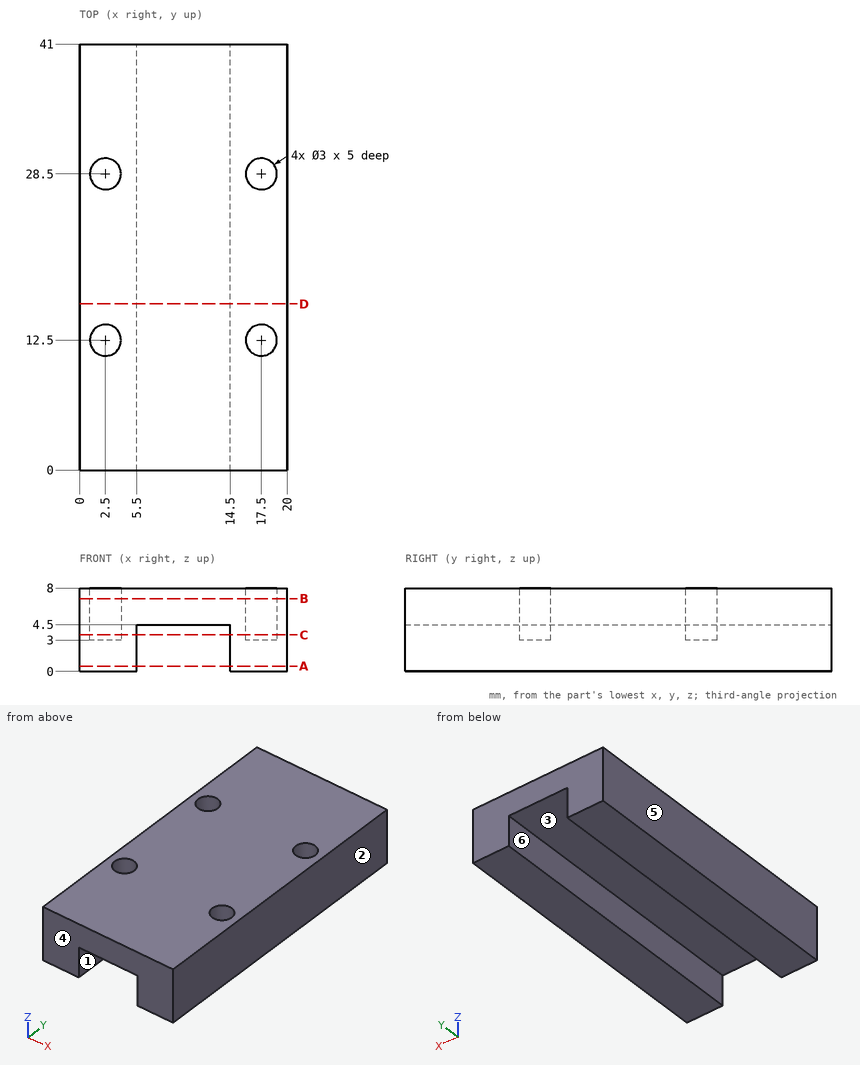
Part print with two shaded views. Sizes in mm from the minimum x, y, z corner. A direction names the side the tool comes from. Round coordinates to 2 decimals unless told otherwise and drop trailing zeros. Order: outer loops, then holes, each group sorted by start corner. A loop starts at its lowest first (then second) coordinate and runs counter-clockwise, first axis right, second up. Notation, with made-up numbers: M -26,71.25 L -22,71.25 A17 cw -22,91.25 Z; hole C 41.25,86.25 d6. An arc over 180 degrees is marked long. Answer in a Markdown table with one row per item. Add a question column.
Q1. Pin check, flat tips, straight feed: pin 1 (1.5 mm diameter, centred on x = 17, y = 28.5, fed in from +Z); pin 2 (1 mm diameter, centred on x = 13, z = 2, fed in from -Y); pin 3 (7 mm diameter, centred on x = 10, y = 15, fed in from -Z). Stop position of each tip, or through.
Q2. Cut at D-D on y = 16. Give the cut face in (x, z), and give its area (4 significant figures).
Q3. Mould opens along X. For the marked faces 3, 4, 5 and 6 say: +X half, -X half, draft (parallel to the pull), parting line (faces both ways), or undercut.
Q4. Cut at B-B on z = 7. Give the cut face in (x, y), and give its area (3 significant figures).
Q5. 3-axis set-ups, long thin cutter, end or side, ignore diameter. For the marked faces 1 and 2: which of +Z, -Z, +X, -X, +Y, -Y reach the whole face in a straight line?
Q6. Cut at C-C on z = 3.5. Give the cut face in (x, y), and give its area (3 significant figures).
Q7. Wall check: L1, parallel to Y at x = 17.5, z = 4.25; L2, parallel to X at y = 25, z = 3; L3, parallel to Y at x = 2, z = 6.5. Give the ranges that are in metal, low to high. Write a range as from..to.
Q8. Cut at A-A on z = 0.5. Give the cut face in (x, y), and give its area (3 significant figures).
Established:
| question | item | result |
|---|---|---|
| 1 | pin 1 | stops at z = 3 |
| 1 | pin 2 | passes through |
| 1 | pin 3 | stops at z = 4.5 |
| 2 | outline | M 0,0 L 5.5,0 L 5.5,4.5 L 14.5,4.5 L 14.5,0 L 20,0 L 20,8 L 0,8 Z |
| 2 | area | 119.5 mm2 |
| 3 | face 3 | undercut |
| 3 | face 4 | draft |
| 3 | face 5 | -X half |
| 3 | face 6 | undercut |
| 4 | outline | M 0,0 L 20,0 L 20,41 L 0,41 Z; hole C 2.5,12.5 d3; hole C 2.5,28.5 d3; hole C 17.5,12.5 d3; hole C 17.5,28.5 d3 |
| 4 | area | 792 mm2 |
| 5 | face 1 | -Z, +Y, -Y |
| 5 | face 2 | +Z, -Z, +X, +Y, -Y |
| 6 | outline | M 0,0 L 5.5,0 L 5.5,41 L 0,41 Z; M 14.5,0 L 20,0 L 20,41 L 14.5,41 Z; hole C 2.5,12.5 d3; hole C 2.5,28.5 d3; hole C 17.5,12.5 d3; hole C 17.5,28.5 d3 |
| 6 | area | 423 mm2 |
| 7 | L1 | y = 0..11, 14..27, 30..41 |
| 7 | L2 | x = 0..5.5, 14.5..20 |
| 7 | L3 | y = 0..11.09, 13.91..27.09, 29.91..41 |
| 8 | outline | M 0,0 L 5.5,0 L 5.5,41 L 0,41 Z; M 14.5,0 L 20,0 L 20,41 L 14.5,41 Z |
| 8 | area | 451 mm2 |
